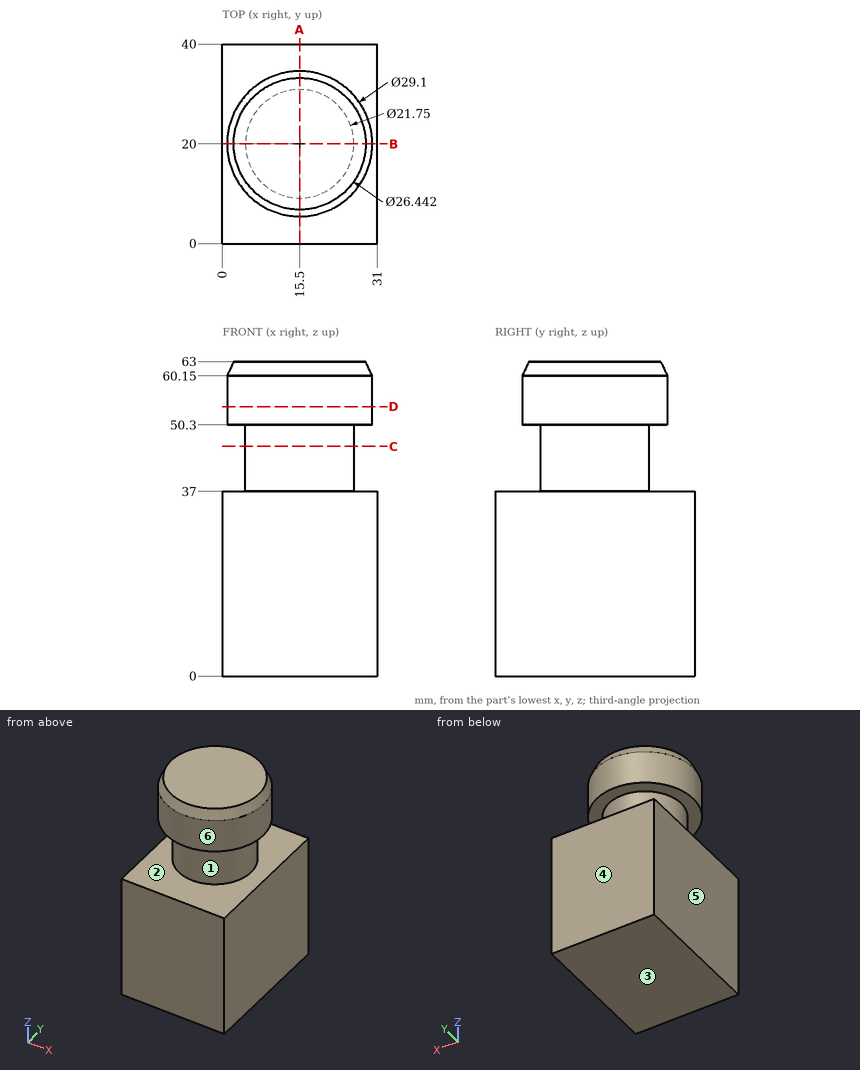
Geometry check sheet. Reference: drawing and pictorial views, mm from the part's lowest x, y, z. A direction names the side the tool comes from. Round coordinates to 2 decimals unless told otherwise and drop trailing zeros. Write each loop counter-clockwise with the first axis right and the second up, starting at its lowest first coordinate (ties: lowest second). Pieces come first, ordered by that corner, then holes.
1. Section check B-B on y = 20. Enter the section's corners in (x, z) (3 decimals), plus the area to 3 significant figures.
2. Scan lines: L1, parallel to Z at x = 26, y = 25; L2, parallel to Z at x = 4, y = 27.5; L3, parallel to Z at x = 26.5, y = 38. Record each from-to range of solid material in increasing order.
3. Access from +Z, -Z, +X, -X, +Y, -Y to the whole of each face (thin tool, end or side, straight path). Record for the marked faces 5 and 6.
4. Section check A-A on x = 15.5. Enter the section's corners in (y, z) (3 decimals).
5. Section check C-C on z = 46. Enter the section's corners in (x, y) (3 decimals).
6. Gauge pin test, flat ends, axial feed: P1, Ø12, axis at x = 17, z = 56, coming from the -Y side; P2, Ø4, axis at y = 14, z = 44, coming from the -X side; P3, Ø2, axis at y = 10, z = 41, coming from the -X side. Record the tip position at first contact, or that the pin passes through.
7. Section check D-D on z = 54. Enter the section's corners in (x, y), plus the area to 3 significant figures.
8. Draft check along Z on the marked faces 1, 2, 3 and 4. Enter one of: +Z half, -Z half, draft (parallel to the pull), parting line (faces both ways), or undercut.
Answer:
1. outline: (0, 0) - (31, 0) - (31, 37) - (26.375, 37) - (26.375, 50.3) - (30.05, 50.3) - (30.05, 60.15) - (28.721, 63) - (2.279, 63) - (0.95, 60.15) - (0.95, 50.3) - (4.625, 50.3) - (4.625, 37) - (0, 37) - close
1. area: 1,800 mm2
2. L1: z = 0 to 37, 50.3 to 63
2. L2: z = 0 to 37, 50.3 to 61.91
2. L3: z = 0 to 37
3. face 5: +Z, -Z, -X, +Y, -Y
3. face 6: +Z
4. outline: (0, 0) - (40, 0) - (40, 37) - (30.875, 37) - (30.875, 50.3) - (34.55, 50.3) - (34.55, 60.15) - (33.221, 63) - (6.779, 63) - (5.45, 60.15) - (5.45, 50.3) - (9.125, 50.3) - (9.125, 37) - (0, 37) - close
5. outline: circle Ø21.75 at (15.5, 20)
6. P1: stops at y = 5.45
6. P2: stops at x = 5.39
6. P3: stops at x = 9.4
7. outline: circle Ø29.1 at (15.5, 20)
7. area: 665 mm2
8. face 1: undercut
8. face 2: undercut
8. face 3: -Z half
8. face 4: draft
